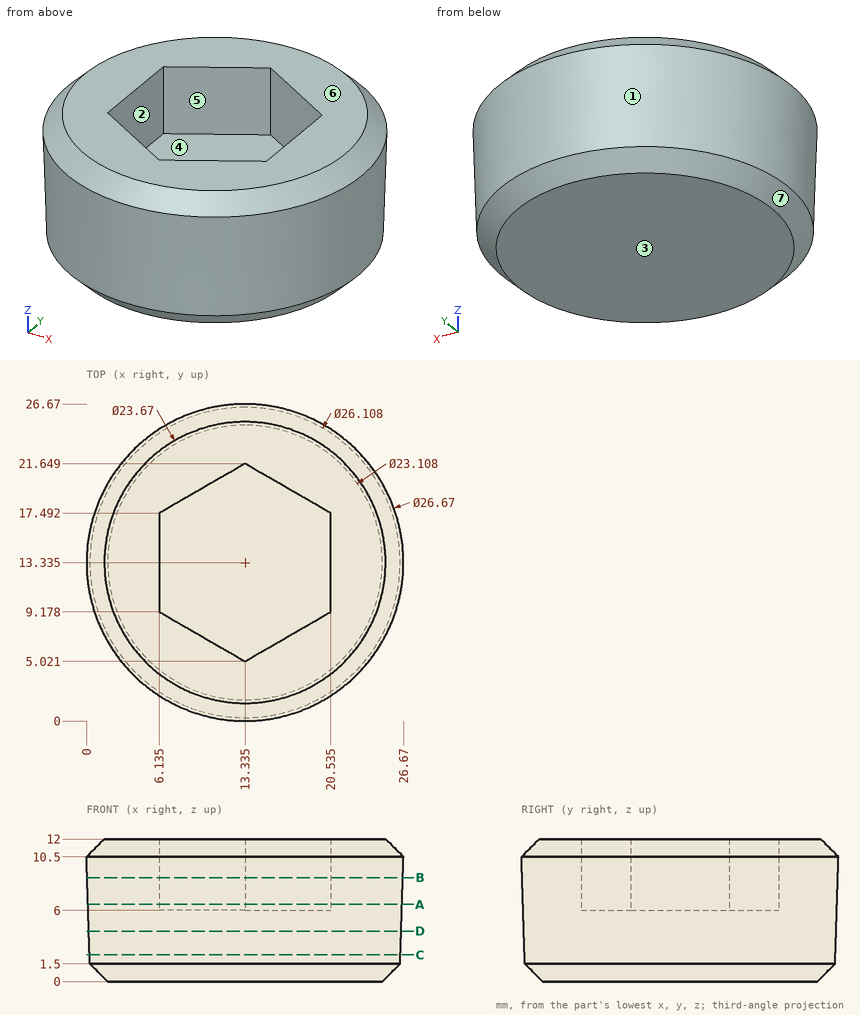
The figure shows three views and two pictorial views of one solid part (mm, origin at its lowest corner). Answer the questions. A direction names the side the tool comes from. Round coordinates to 2 decimals unless told otherwise and drop trailing zeros. Loops run counter-clockwise (first coordinate to the right, second up) from the corner with the lowest first, then second, coordinate; pieces in that order, holes last. Notation, with made-up numbers: M 25.5,56 L 32.5,56 A4 ccw 32.5,61 Z; hole C -40,-15.75 d3. An arc over 180 degrees is marked long. Return JSON: item names as keys, results as strings.
Q1. Find section B-B, the plane z = 8.75. Determine the outline of the cut face in (x, y) (1 decimal), plus the area to 4 significant figures.
Results list:
{"outline": "C 13.3,13.3 d26.6; hole M 6.1,9.2 L 13.3,5 L 20.5,9.2 L 20.5,17.5 L 13.3,21.6 L 6.1,17.5 Z", "area": "374.5 mm2"}
Q2. Which of the six approach directions +Z, -Z, +X, -X, +Y, -Y give full straight-line access (tool end or side, diameter ignored) to the marked faces 1, 2 and 3?
Results list:
{"face 1": "-Z", "face 2": "+Z", "face 3": "-Z, +X, -X, +Y, -Y"}
Q3. Find section D-D, the plane z = 4.25. Determine the outline of the cut face in (x, y) (1 decimal), plus the area to 3 significant figures.
Results list:
{"outline": "C 13.3,13.3 d26.3", "area": "542 mm2"}
Q4. Find the intervals of material crossed by line 1 along X through (y, z) = (10.75, 7.75) (1 decimal); line 2 along Y through (x, z) = (20, 7); line 3 along Z through (x, y) = (16.25, 14.75), in increasing order. Write a range as from..to.
Results list:
{"line 1": "x = 0.3..6.1, 20.5..26.3", "line 2": "y = 1.91..8.87, 17.8..24.76", "line 3": "z = 0..6"}
Q5. Find section A-A, the plane z = 6.5. Determine the outline of the cut face in (x, y) (1 decimal), plus the area to 3 significant figures.
Results list:
{"outline": "C 13.3,13.3 d26.4; hole M 6.1,9.2 L 13.3,5 L 20.5,9.2 L 20.5,17.5 L 13.3,21.6 L 6.1,17.5 Z", "area": "369 mm2"}
Q6. The mould has two halves that part along Y. Classify the marked faces 4, 5, 6 and 7: released by +Y, released by -Y, zero draft, split by the parting line, or undercut.
Results list:
{"face 4": "undercut", "face 5": "undercut", "face 6": "zero draft", "face 7": "split by the parting line"}
Q7. Find section C-C, the plane z = 2.25. Determine the outline of the cut face in (x, y) (1 decimal), plus the area to 3 significant figures.
Results list:
{"outline": "C 13.3,13.3 d26.2", "area": "537 mm2"}
Q8. Each of these flat-tipped pins is pushed along its axis until it touches: pin 1 Ø1.8 at (y, z) = (14, 8.5) entering from +X; pin 2 Ø10 at (x, y) = (18, 5) entering from -Z; pin 3 Ø2 at (y, z) = (15.5, 5.5) entering from -X; pin 4 Ø4.5 at (x, y) = (12.5, 13) entering from +Z. Where does it stop, or does it pass through?
Results list:
{"pin 1": "stops at x = 26.63", "pin 2": "stops at z = 0", "pin 3": "stops at x = 0.2", "pin 4": "stops at z = 6"}
